Build history of the part. All positions in model axes, mm. Round coordinates to 2 decimals unless told otherwise and drop trailing zeros. Write each loop counter-clockwise with the first axis right and the second up, starting at its lowest first coordinate (ties: lowest second). Pieces come first, ordered by that corner, then holes. Notation, with made-up numbers: (-19, 61.25) - (21, 61.25) arc R31 ccw to (21, 91.25) - close; hole circle Ø2 at (-2, 9.5). An arc over 180 degrees is marked (long way). Write each question's results on one line, items separated by ' | '.
Autodesk Inventor part; units mm, degrees
ref_plane "YZ Plane" through (0, 0, 0) normal (1, 0, 0) x (0, 1, 0)
ref_plane "XZ Plane" through (0, 0, 0) normal (0, 1, 0) x (-1, 0, 0)
ref_plane "XY Plane" through (0, 0, 0) normal (0, 0, 1) x (1, 0, 0)
sketch "Sketch1" plane through (0, 0, 0) normal (0, 1, 0) x (-1, 0, 0)
  line L0 (0, 0) -> (0, -200)
  line L1 (0, -200) -> (90, -200)
  line L2 (90, -200) -> (90, 0)
  line L3 (90, 0) -> (0, 0)
  line L4 (45, -200) -> (45, -188)
  line L5 (45, -188) -> (56.125, -188)
  line L6 (56.125, -188) -> (56.125, -162)
  line L7 (56.125, -162) -> (33.875, -162)
  line L8 (33.875, -162) -> (33.875, -188)
  line L9 (33.875, -188) -> (45, -188)
  line L10 (45, -150) -> (56.125, -150)
  line L11 (56.125, -150) -> (56.125, -124)
  line L12 (56.125, -124) -> (33.875, -124)
  line L13 (33.875, -124) -> (33.875, -150)
  line L14 (33.875, -150) -> (45, -150)
  line L15 (45, -112) -> (56.125, -112)
  line L16 (56.125, -112) -> (56.125, -86)
  line L17 (56.125, -86) -> (33.875, -86)
  line L18 (33.875, -86) -> (33.875, -112)
  line L19 (33.875, -112) -> (45, -112)
  circle A0 centre (86, -4) radius 2.1
  circle A1 centre (86, -100) radius 2.1
  circle A2 centre (86, -196) radius 2.1
  circle A3 centre (4, -4) radius 2.1
  circle A4 centre (4, -100) radius 2.1
  circle A5 centre (4, -196) radius 2.1
  dimension "d0" = 200
  dimension "d1" = 90
  dimension "d2" = 200
  dimension "d3" = 12
  dimension "d4" = 11.125
  dimension "d5" = 26
  dimension "d6" = 22.25
  dimension "d7" = 26
  dimension "d9" = 11.125
  dimension "d10" = 26
  dimension "d11" = 22.25
  dimension "d12" = 26
  dimension "d14" = 11.125
  dimension "d15" = 26
  dimension "d16" = 22.25
  dimension "d17" = 26
  dimension "d23" = 4.2
  dimension "d25" = 4.2
extrude "Extrusion1" add sketch "Sketch1" against normal blind 2
properties part number "Cover Rev 4"
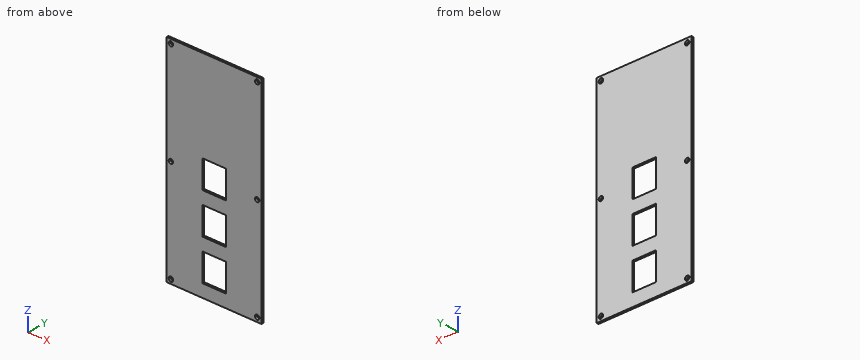
(1) Drill centre lines: probe 1 along Z at (x, y) = (-4, -1); probe 2 along Z at (x, y) = (-47.5, -0.1); probe 3 along X at (y, z) = (-1.4, -196). Where is each one in solid material? Low to high. Write a range as [from, to].
Worked answers:
probe 1: z = [-200, -198.1], [-193.9, -102.1], [-97.9, -6.1], [-1.9, 0] | probe 2: z = [-200, -188], [-162, -150], [-124, -112], [-86, 0] | probe 3: x = [-90, -88.1], [-83.9, -6.1], [-1.9, 0]
(2) Flat gauge pin, fed straight in: pin 1 Ø3.5 at (x, z) = (-4, -4) entering from -Y. Where does the tip first touch, or does it go through?
Worked answers:
pin 1: passes through
(3) Slice it at A-A, the plane z = -4. Write the cut outline in (x, y), and give its area (3 significant figures).
Worked answers:
outline: (-90, -2) - (-88.1, -2) - (-88.1, 0) - (-90, 0) - close; (-83.9, -2) - (-6.1, -2) - (-6.1, 0) - (-83.9, 0) - close; (-1.9, -2) - (0, -2) - (0, 0) - (-1.9, 0) - close | area: 163 mm2
(4) Slice it at B-B, the plane x = -4. Write the cut outline in (y, z).
Worked answers:
outline: (-2, -200) - (0, -200) - (0, -198.1) - (-2, -198.1) - close; (-2, -193.9) - (0, -193.9) - (0, -102.1) - (-2, -102.1) - close; (-2, -97.9) - (0, -97.9) - (0, -6.1) - (-2, -6.1) - close; (-2, -1.9) - (0, -1.9) - (0, 0) - (-2, 0) - close
(5) Slice it at C-C, the plane y = -1.6. State how many separate pieces and enclosed holes the cut face has, and give its area (3 significant figures).
Worked answers:
separate pieces: 1 | enclosed holes: 9 | area: 16,200 mm2
(6) Slice it at D-D, the plane z = -136. Write the cut outline in (x, y) (3 decimals).
Worked answers:
outline: (-90, -2) - (-56.125, -2) - (-56.125, 0) - (-90, 0) - close; (-33.875, -2) - (0, -2) - (0, 0) - (-33.875, 0) - close
